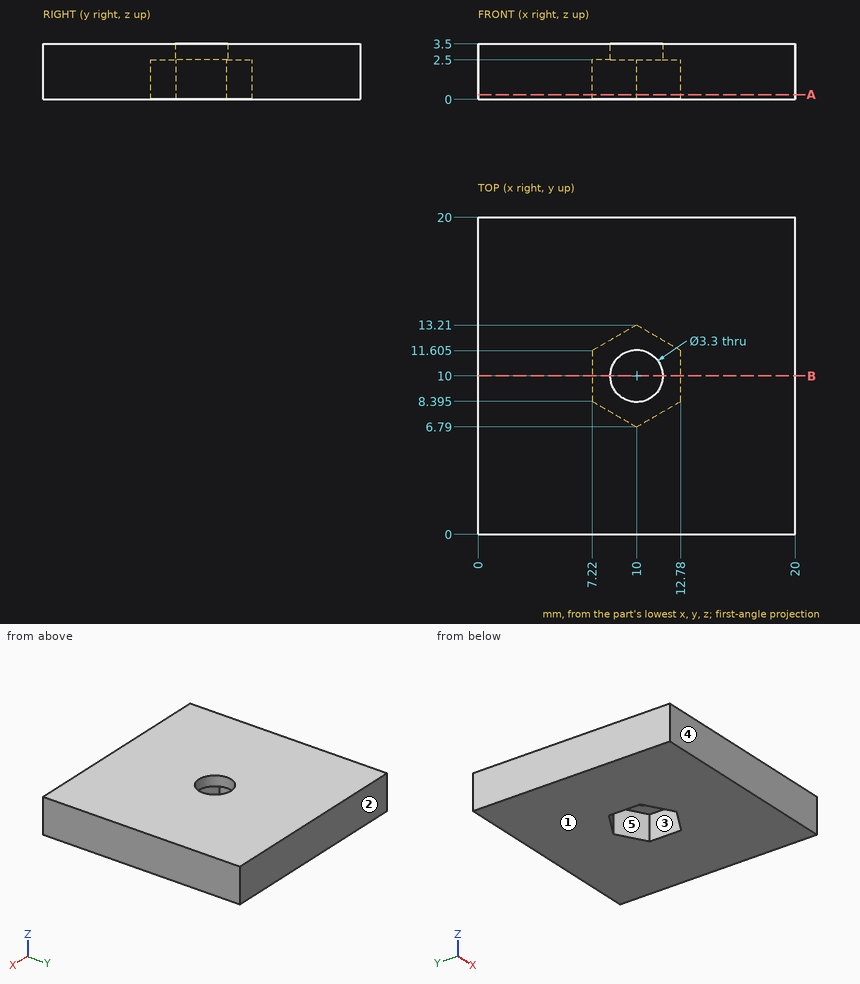
Design review of the part shown in the three views and the two pictorial views. Dimensions are in mm from the part's minimum x, y and z. A direction names the side the tool comes from. Coordinates: 2 decimals unless noted, no trailing zeros. Write each loop counter-clockwise with the first axis right and the second up, starting at its lowest first coordinate (ties: lowest second). Pieces come first, ordered by that corner, then holes.
(1) Tool access review of the marked faces 4 and 5: name each direction out of +Z, -Z, +X, -X, +Y, -Y from which nothing blocks a thin tool from reaching the whole face with its end or side.
(2) Wall thickness on probe 1 along Y at (x, z) = (10, 3.35); probe 2 along Z at (x, y) = (9.75, 7.25); probe 3 along Y at (x, z) = (11.5, 1.25): over which ranges is each line inside the solid? List them lowest first.
(3) Add section B-B on y = 10. Give the boundary of the cut face in (x, z).
(4) The part is to be moulded in two halves that separate along Y. For the marked faces 1, 2 and 3, say which applies: +Y half, -Y half, draft (parallel to the pull), parting line (faces both ways), or undercut.
(5) Add section A-A on z = 0.3. Give the boundary of the cut face in (x, y) (3 decimals), then the cut area to 3 significant figures.
(6) For pin 1 Ø2 at (y, z) = (10.5, 1.5) entering from -X; pin 2 Ø3 at (x, y) = (9.5, 9) entering from -Z; pin 3 Ø2.5 at (x, y) = (10, 10) entering from -Z, all flat-tipped, find the tip position at first contact; note any pin that passes through.
Answer sheet:
1. face 4: +Z, -Z, +X, -X, -Y
1. face 5: -Z
2. probe 1: y = 0 to 8.35, 11.65 to 20
2. probe 2: z = 2.5 to 3.5
2. probe 3: y = 0 to 7.66, 12.34 to 20
3. outline: (0, 0) - (7.22, 0) - (7.22, 2.5) - (8.35, 2.5) - (8.35, 3.5) - (0, 3.5) - close; (11.65, 2.5) - (12.78, 2.5) - (12.78, 0) - (20, 0) - (20, 3.5) - (11.65, 3.5) - close
4. face 1: draft
4. face 2: +Y half
4. face 3: undercut
5. outline: (0, 0) - (20, 0) - (20, 20) - (0, 20) - close; hole (7.22, 8.395) - (10, 6.79) - (12.78, 8.395) - (12.78, 11.605) - (10, 13.21) - (7.22, 11.605) - close
5. area: 373 mm2
6. pin 1: stops at x = 0
6. pin 2: stops at z = 2.5
6. pin 3: passes through
